from build123d import *

# Parameters (mm, degrees)
ESQUISSE1_R             = 46
BOSS_EXTRU_1_DEPTH      = 4
ESQUISSE2_R             = 8
ENL_V_MAT_EXTRU_1_DEPTH = 4.5
ENL_V_MAT_EXTRU_2_DEPTH = 2


with BuildPart() as part:
    # Esquisse1 → Boss.-Extru.1 (new body)
    with BuildSketch(Plane(origin=(0, 0, 0), x_dir=(1, 0, 0), z_dir=(0, 1, 0))):
        with Locations(Location((0, 0, 0), (0, 0, 270))):
            Circle(ESQUISSE1_R)
    extrude(amount=BOSS_EXTRU_1_DEPTH)

    # Esquisse2 → Enlèv. mat.-Extru.1 (cut)
    with BuildSketch(Plane(origin=(0, 4, 0), x_dir=(1, 0, 0), z_dir=(0, 1, 0))):
        with Locations(Location((0, 0, 0), (0, 0, 270))):
            Circle(ESQUISSE2_R)
    extrude(amount=-ENL_V_MAT_EXTRU_1_DEPTH, mode=Mode.SUBTRACT)

    # Esquisse3 → Enlèv. mat.-Extru.2 (cut)
    with BuildSketch(Plane(origin=(0, 0, 0), x_dir=(-1, 0, 0), z_dir=(0, -1, 0))):
        with BuildLine():
            ThreePointArc((0, -32), (22.627416998, -22.627416998), (32, 0))
            ThreePointArc((32, 0), (31, 0.918210565), (30, 0))
            ThreePointArc((30, 0), (0, -30), (-30, 0))
            ThreePointArc((-30, 0), (-31, 1), (-32, 0))
            ThreePointArc((-32, 0), (-22.627416998, -22.627416998), (0, -32))
        make_face()
    extrude(amount=-ENL_V_MAT_EXTRU_2_DEPTH, mode=Mode.SUBTRACT)


solid = part.part
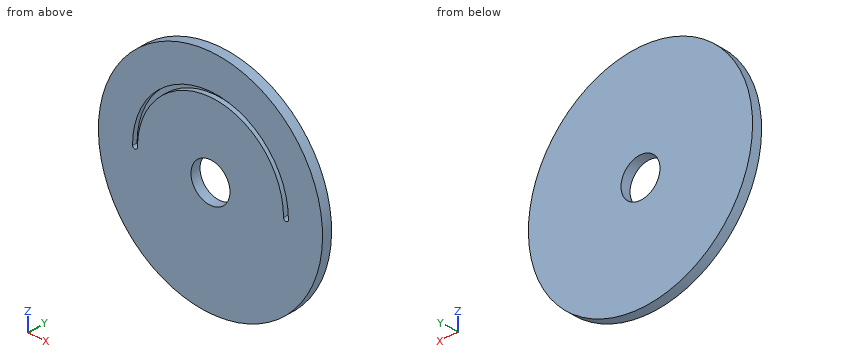
Input: part model. Units: mm. Frame: model coordinates. Coordinates: 2 decimals unless noted, no trailing zeros. Write each loop counter-clockwise with the first axis right and the second up, starting at its lowest first coordinate (ties: lowest second). Pieces come first, ordered by that corner, then holes. Notation, with made-up numbers: M 60.5,63 L 114.5,63 A31 ccw 114.5,92 Z; hole C 56,-32 d11. An arc over 180 degrees is marked long. Answer as a JSON object with one key per item and string values. Group by question number.
(1) Section D-D on z = -37. Output: boundary loops of the cut face in (x, y).
(2) Section C-C on x = -22. Output: boundary loops of the cut face in (y, z).
(3) Contact query for flat-ended pins moving along their axis: P1, Ø5, axis at x = 3.5, z = 28.5, coming from the -Y side; P2, Ø2, axis at y = 3, z = 1, coming from the -X side. Output: stop coordinate, or through.
(4) Section B-B on x = 3. Output: boundary loops of the cut face in (y, z).
(5) Ray query, line 1 along X through (y, z) = (2.35, 0); line 2 along Z through (x, y) = (6, 1.85); line 3 along Z through (x, y) = (4, 0.35). Return the intervals inside material, ascending. Write a range as [from, to].
(6) Section A-A on y = 1. Output: boundary loops of the cut face in (x, z), plus the area to 3 significant figures.
Result set:
{
 "1": {"outline": "M -27.33,0 L 27.33,0 L 27.33,4 L -27.33,4 Z"},
 "2": {"outline": "M 0,-40.4 L 4,-40.4 L 4,40.4 L 0,40.4 L 0,23.24 L 2,23.24 L 2,20.4 L 0,20.4 Z"},
 "3": {"P1": "stops at y = 0", "P2": "stops at x = -46"},
 "4": {"outline": "M 0,-45.9 L 4,-45.9 L 4,-7.42 L 0,-7.42 Z; M 0,7.42 L 4,7.42 L 4,45.9 L 0,45.9 L 0,31.86 L 2,31.86 L 2,29.85 L 0,29.85 Z"},
 "5": {"line 1": "x = [-46, -8], [8, 46]", "line 2": "z = [-45.61, -5.29], [5.29, 29.39], [31.43, 45.61]", "line 3": "z = [-45.83, -6.93], [6.93, 29.73], [31.75, 45.83]"},
 "6": {"outline": "C 0,0 d92; hole M -32,0 A1 ccw -30,0 A30 cw 30,0 A1 ccw 32,0 A32 ccw Z; hole C 0,0 d16", "area": "6,250 mm2"}
}
